The listing builds one solid part. Answer for the finished solid, in the listing's coordinates (mm). A direction names the side the tool comes from. Round coordinates to 2 decimals unless told otherwise and drop trailing zeros. Order: outer loops, then holes, each group sorted by start corner. A loop starts at its lowest first (then second) coordinate and runs counter-clockwise, first axis right, second up. Notation, with made-up numbers: M 87.5,25 L 115.5,25 A12 ccw 115.5,33 Z; hole C 3.5,55 d9. An arc over 180 degrees is marked long. Put each result on its own line as item: value. Start each with the question number.
1. The part is cut by section A-A (y = 1). Give the vertices of the cut face in (x, z).
2. Which of the six approach directions +Z, -Z, +X, -X, +Y, -Y give full straight-line access (tool end or side, diameter ignored) to faces 5 (the face through (0, 15, -1)), 6 (the face through (-14.699, -14.715, -1.479)), 7 (the face through (9, -15, -1))?
3. The part is cut by section B-B (x = 6.5). Give the vertices of the cut face in (y, z).
4. The part is cut by section C-C (z = 0.9). Give the vertices of the cut face in (x, y).
5. Consider line 1 (X direction, y = -0.5, z = 1.7); line 2 (X direction, y = 8, z = -0.65). Determine where each line is inside the solid, lowest interval first.
6. The mould has two halves that part along X. Classify faces 1 (the face through (-15, 0, -1)), 2 (the face through (-1.5, -6, 0)), 3 (the face through (0, 17, 0)), 4 (the face through (3.519, -6, -1)): +X half, -X half, draft (parallel to the pull), parting line (faces both ways), or undercut.
7. Each of these flat-tipped pins is pushed along its axis until it touches: pin 1 Ø0.9 at (y, z) = (3, -1.5) entering from -X; pin 2 Ø0.9 at (y, z) = (1, -2) entering from +X; pin 3 Ø3 at (x, z) = (-11.5, -2) entering from +Y. Where does it stop, or does it pass through?
from build123d import *

# Parameters (mm, degrees)
F1_DEPTH = 2
F3_DEPTH = 3


with BuildPart() as f1:
    # F0 (on Top) → F1 (new body)
    with BuildSketch(Plane.XY):
        with BuildLine():
            Line((17, 19), (-17, 19))
            ThreePointArc((-17, 19), (-18.414214, 18.414214), (-19, 17))
            Line((-19, 17), (-19, -17))
            ThreePointArc((-19, -17), (-18.414214, -18.414214), (-17, -19))
            Line((-17, -19), (-1.5, -19))
            Line((-1.5, -19), (-1.5, 6.522064))
            Line((-1.5, 6.522064), (1.5, 6.522064))
            Line((1.5, 6.522064), (1.519474, 6.522064))
            Line((1.519474, 6.522064), (3.519474, 6.522064))
            Line((3.519474, 6.522064), (3.519474, -19))
            Line((3.519474, -19), (17, -19))
            ThreePointArc((17, -19), (18.414214, -18.414214), (19, -17))
            Line((19, -17), (19, 17))
            ThreePointArc((19, 17), (18.414214, 18.414214), (17, 19))
        make_face()
    extrude(amount=F1_DEPTH)

    # F2 (on face) → F3 (join)
    with BuildSketch(Plane(origin=(0, 0, 0), x_dir=(1, 0, 0), z_dir=(0, 0, -1))):
        with BuildLine():
            Line((-1.5, 15), (-14, 15))
            ThreePointArc((-14, 15), (-14.707107, 14.707107), (-15, 14))
            Line((-15, 14), (-15, -14))
            ThreePointArc((-15, -14), (-14.707107, -14.707107), (-14, -15))
            Line((-14, -15), (14, -15))
            ThreePointArc((14, -15), (14.707107, -14.707107), (15, -14))
            Line((15, -14), (15, 14))
            ThreePointArc((15, 14), (14.707107, 14.707107), (14, 15))
            Line((14, 15), (3.519474, 15))
            Line((3.519474, 15), (3.519474, -6.522064))
            Line((3.519474, -6.522064), (-1.5, -6.522064))
            Line((-1.5, -6.522064), (-1.5, 15))
        make_face()
    extrude(amount=F3_DEPTH)


solid = f1.part
Resolved:
1. outline: M -19,0 L -15,0 L -15,-3 L -1.5,-3 L -1.5,2 L -19,2 Z; M 3.52,-3 L 15,-3 L 15,0 L 19,0 L 19,2 L 3.52,2 Z
2. face 5: -Z, +X, -X, +Y
2. face 6: -Z, -X, -Y
2. face 7: -Z, +X, -X, -Y
3. outline: M -19,0 L -15,0 L -15,-3 L 15,-3 L 15,0 L 19,0 L 19,2 L -19,2 Z
4. outline: M -19,-17 A2 ccw -17,-19 L -1.5,-19 L -1.5,6.52 L 3.52,6.52 L 3.52,-19 L 17,-19 A2 ccw 19,-17 L 19,17 A2 ccw 17,19 L -17,19 A2 ccw -19,17 Z
5. line 1: -19 to -1.5, 3.52 to 19
5. line 2: -15 to 15
6. face 1: -X half
6. face 2: undercut
6. face 3: draft
6. face 4: undercut
7. pin 1: x = -15
7. pin 2: x = 15
7. pin 3: y = 15
